The listing builds one solid part. Answer for the finished solid, in the listing's coordinates (mm). A direction names the side the tool comes from. Round coordinates to 2 decimals unless told otherwise and drop trailing zeros. Loops run counter-clockwise (first coordinate to the right, second up) from the corner with the lowest first, then second, coordinate; pieces in that order, holes last. Notation, with made-up numbers: (13.5, 19.5) -> (44.5, 19.5) arc R21 cw to (44.5, 36.5) -> close; hole circle Ø8 at (82.5, 30.5). An arc over 180 degrees is marked (long way). Use a Markdown table: item, result. Add a question column.
Q1. Section C-C on z = 32 is taken. Give the vertices of the cut face in (x, y).
Q2. Consider line 1 (Z direction, x = 12.5, y = 10); line 2 (Y direction, x = 13, z = 45); line 3 (Z direction, x = 10, y = 1.5). Determine where each line is inside the solid, lowest interval first.
Q3. Which of the six approach directions +Z, -Z, +X, -X, +Y, -Y give full straight-line access (tool end or side, diameter ignored) to faces 1 (the flat face through (9, -2, 80)), 2 (the flat face through (9, 4.8, 39)), 3 (the flat face through (4.2, 3, 47))?
Q4. Given pin 1 Ø3.5 at (x, y) = (8, -2) entering from -Z; pin 2 Ø5 at (x, z) = (6, 64.5) entering from +Y; pin 3 Ø3 at (x, z) = (11, 37) entering from -Y, each flat-ended and moving along its own axis, determine where each tip first touches the part or whether it passes through.
Q5. Section A-A on x = 8.75 is taken. Give the vertices of the cut face in (y, z).
Q6. Section B-B on y = 0 is taken. Give the vertices of the cut face in (x, z).
Autodesk Inventor part; units mm, degrees
ref_plane "YZ Plane" through (0, 0, 0) normal (1, 0, 0) x (0, 1, 0)
ref_plane "XZ Plane" through (0, 0, 0) normal (0, 1, 0) x (-1, 0, 0)
ref_plane "XY Plane" through (0, 0, 0) normal (0, 0, 1) x (1, 0, 0)
sketch "Sketch1" plane through (0, 0, 0) normal (0, 0, 1) x (1, 0, 0)
  arc A0 (16, 5) -> (14, 7) centre (14, 5) ccw
  line L0 (14, 7) -> (8, 7)
  arc A1 (6, 9) -> (8, 7) centre (8, 9) ccw
  line L1 (6, 9) -> (6, 25.5)
  arc A2 (6, 25.5) -> (4, 27.5) centre (4, 25.5) ccw
  line L2 (4, 27.5) -> (-14, 27.5)
  arc A3 (-14, 27.5) -> (-16, 25.5) centre (-14, 25.5) ccw
  line L3 (-16, 25.5) -> (-16, 20.5)
  line L4 (-16, 20.5) -> (4, 20.5)
  line L5 (4, 20.5) -> (4, 5)
  line L6 (4, 5) -> (14, 5)
  line L7 (14, 5) -> (14, -15)
  line L8 (14, -15) -> (4, -15)
  line L9 (4, -15) -> (4, -20.5)
  line L10 (4, -20.5) -> (-16, -20.5)
  line L11 (-16, -20.5) -> (-16, -25.5)
  arc A4 (-16, -25.5) -> (-14, -27.5) centre (-14, -25.5) ccw
  line L12 (-14, -27.5) -> (4, -27.5)
  arc A5 (4, -27.5) -> (6, -25.5) centre (4, -25.5) ccw
  line L13 (6, -25.5) -> (6, -19)
  arc A6 (8, -17) -> (6, -19) centre (8, -19) ccw
  line L14 (8, -17) -> (14, -17)
  arc A7 (14, -17) -> (16, -15) centre (14, -15) ccw
  line L15 (16, -15) -> (16, 5)
  circle A8 centre (-10.2273, -23.9687) radius 0.75
  circle A9 centre (-0.7, 24) radius 0.75
  circle A10 centre (-10.2, 24) radius 0.75
  circle A11 centre (-0.7, -24) radius 0.75
  line L16 (14, 5) -> (4, 5)
  line L17 (4, 5) -> (4, 2)
  line L18 (4, 2) -> (14, 2)
  line L19 (14, 2) -> (14, 5)
  point P0 (0, 0)
extrude "Extrusion1" add sketch "Sketch1" along normal blind 80 contours L6 L7 L18 L17
sketch "Sketch2" plane through (0, 0, 80) normal (0, 0, 1) x (1, 0, 0)
  line L0 (14, 2) -> (14, 5)
  line L1 (14, 5) -> (4, 5)
  line L2 (4, 5) -> (4, 2)
  line L3 (4, 2) -> (14, 2)
  line L4 (14, 2) -> (4, 2)
  line L5 (4, 2) -> (4, -6)
  line L6 (4, -6) -> (14, -6)
  line L7 (14, -6) -> (14, 2)
  line L8 (14, 5) -> (4, 5)
  line L9 (4, 5) -> (4, 11)
  line L10 (4, 11) -> (14, 11)
  line L11 (14, 11) -> (14, 5)
  point P0 (0, 0)
  dimension "d2" = 8
  dimension "d3" = 6
extrude "Extrusion2" add sketch "Sketch2" along normal blind 3
chamfer "Chamfer1" distance 1 angle 45 2 edges at (9, 2, 80) (9, 5, 80)
thicken "Thicken1" operation add thickness 0.2 both sides no extend neighbours yes toward (1, 0, 0) faces at (4, 4, 26.3333) (7.3333, 2, 26.3333) (14, 3, 26.3333) (10.6667, 5, 26.3333)
properties part number "fence"
Checked values:
| question | item | result |
|---|---|---|
| 1 | outline | (4.2, 2.2) -> (13.8, 2.2) -> (13.8, 4.8) -> (4.2, 4.8) -> close |
| 2 | line 1 | z = 80 to 83 |
| 2 | line 2 | y = 2.2 to 4.8 |
| 2 | line 3 | z = 79.5 to 83 |
| 3 | face 1 | -Z, +X, -X, -Y |
| 3 | face 2 | -Z, +X, -X, +Y |
| 3 | face 3 | +Z, -Z, -X, +Y, -Y |
| 4 | pin 1 | stops at z = 80 |
| 4 | pin 2 | stops at y = 4.8 |
| 4 | pin 3 | stops at y = 2.2 |
| 5 | outline | (-6, 80) -> (1, 80) -> (2.2, 78.8) -> (2.2, 0) -> (4.8, 0) -> (4.8, 78.8) -> (6, 80) -> (11, 80) -> (11, 83) -> (-6, 83) -> close |
| 6 | outline | (4.2, 80) -> (13.8, 80) -> (13.8, 83) -> (4.2, 83) -> close |
